Autodesk Inventor part; units mm, degrees
ref_plane "YZ Plane" through (0, 0, 0) normal (1, 0, 0) x (0, 1, 0)
ref_plane "XZ Plane" through (0, 0, 0) normal (0, 1, 0) x (-1, 0, 0)
ref_plane "XY Plane" through (0, 0, 0) normal (0, 0, 1) x (1, 0, 0)
sketch "Skizze10" plane through (0, 0, 0) normal (1, 0, 0) x (0, 1, 0)
  arc A0 (0, -9.6) -> (0, 9.6) centre (0, 0) ccw
  line L0 (0, 0) -> (0, -24.5)
  line L1 (0, 0) -> (0, 24.5)
  line L2 (0, 15.79) -> (24.9524, 15.79) construction
  line L3 (-4.9905, 0) -> (29.9429, 0)
  line L4 (0, -19.91) -> (23.7326, -19.91) construction
  line L5 (0, 24.5) -> (9.5, 24.5)
  line L6 (9.5, 24.5) -> (9.5, 10.2835)
  arc A1 (9.5, -10.2835) -> (9.5, 10.2835) centre (0, 0) ccw
  line L7 (9.5, -10.2835) -> (9.5, -24.5)
  line L8 (0, -24.5) -> (9.5, -24.5)
  point P0 (0, 9.6)
  point P1 (9.5, -19.91)
  point P2 (9.5, 15.79)
  dimension "d79" = 9.6
  dimension "d80" = 24.5
  dimension "d81" = 24.5
  dimension "d82" = 15.79
  dimension "d83" = 19.91
  dimension "d84" = 9.5
  dimension "d85" = 14
extrude "Extrusion9" add sketch "Skizze10" along normal mid plane 8.5 contours A0 L3 A1 L7 L8 L0 | A0 L1 L5 L6 A1 L3
sketch "Skizze11" plane through (0, 0, 0) normal (0, 1, 0) x (-1, 0, 0)
  circle A0 centre (0, -19.91) radius 1.7
  circle A1 centre (0, 15.79) radius 1.7
  line L0 (-4.25, -24.5) -> (-4.25, -10.2835)
  line L1 (0, -32.898) -> (0, 25.888)
  point P0 (0, 0)
  dimension "d88" = 15.79
  dimension "d89" = 19.91
  dimension "d90" = 3.4
  dimension "d91" = 3.4
extrude "Extrusion10" cut sketch "Skizze11" along normal through all
sketch "Skizze12" plane through (0, 0, 0) normal (0, 1, 0) x (-1, 0, 0)
  line L0 (4.25, 9.6) -> (4.25, 24.5)
  line L1 (4.25, 23) -> (-1.05, 23)
  line L2 (-1.05, 23) -> (-1.05, 18.6)
  line L3 (-1.05, 18.6) -> (4.25, 18.6)
  line L4 (4.25, 18.6) -> (4.25, 23)
  line L5 (5.31, 0) -> (-2.11, 0)
  point P0 (0, 0)
  point P1 (4.25, 18.6)
  dimension "d94" = 4.4
  dimension "d95" = 5.3
  dimension "d96" = 18.6
extrude "Extrusion11" cut sketch "Skizze12" along normal blind 3.35
properties part number "Lagerhalter1"
For this review, take the finished solid that the model builds, in its own axes (mm). A direction names the side the tool comes from. Round coordinates to 2 decimals unless told otherwise and drop trailing zeros. Write each loop counter-clockwise with the first axis right and the second up, starting at its lowest first coordinate (ties: lowest second). Pieces come first, ordered by that corner, then holes. Notation, with made-up numbers: M 55,71 L 73,71 A28 ccw 73,89 Z; hole C 54,55.25 d5. An arc over 180 degrees is marked long. Write item = value, one per line. Start each with the question number.
(1) For faces 1 (the face through (-2, 2, 18.6)), 2 (the face through (-4.25, 10, 0)), 3 (the face through (-1, 9.5, 17.5)), 4 (the face through (0, 9.5, -17)), list the 3-axis set-ups (+Z, -Z, +X, -X, +Y, -Y) from which the entire face can be reached by the end or side of a thin tool; tool diameter is ignored.
(2) The part is to be moulded in two halves that separate along X. For faces 5 (the face through (0.2, 4.7, 14.1)), 6 (the face through (-2, 2, 23)), 7 (the face through (4.25, 10, 0)), say which applies: +X half, -X half, draft (parallel to the pull), parting line (faces both ways), or undercut.
(3) For line 1 along X through (y, z) = (3.5, -19.91); line 2 along Z through (x, y) = (0, 3.25); line 3 along Y through (x, z) = (-1.75, -21), list the stretches that pass through material, from the lowest coordinate up.
(4) We need section C-C (z = -19.91). Give the boundary of the cut face in (x, y).
(5) We need section A-A (y = 6.75). Give the boundary of the cut face in (x, z), then the cut area to 3 significant figures.
(6) We need section B-B (x = 0). Give the boundary of the cut face in (y, z), then the cut area to 3 significant figures.
(7) We need section D-D (x = 2.25). Give the boundary of the cut face in (y, z).
(8) Clearance check with flat-ended pins moving along their axes: pin 1 Ø3.5 at (y, z) = (1, 20) entering from -X; pin 2 Ø1.5 at (x, z) = (-1.5, 0.5) entering from -Y; pin 3 Ø2.5 at (x, z) = (2, 18.5) entering from +Y. State where each tip first meets the part, or that it passes through.
Results found:
q1.face_1 = -X, -Y
q1.face_2 = +Z, -Z, -X, +Y, -Y
q1.face_3 = +Z, +X, -X, +Y
q1.face_4 = -Z, +X, -X, +Y
q2.face_5 = undercut
q2.face_6 = draft
q2.face_7 = +X half
q3.line_1 = -4.25 to -1.7, 1.7 to 4.25
q3.line_2 = -24.5 to -21.61, -18.21 to -9.03, 9.03 to 14.09, 17.49 to 18.6, 23 to 24.5
q3.line_3 = 0 to 9.5
q4.outline = M -4.25,0 L -1.7,0 L -1.7,9.5 L -4.25,9.5 Z; M 1.7,0 L 4.25,0 L 4.25,9.5 L 1.7,9.5 Z
q5.outline = M -4.25,-24.5 L 4.25,-24.5 L 4.25,-6.83 L -4.25,-6.83 Z; M -4.25,6.83 L 4.25,6.83 L 4.25,24.5 L -4.25,24.5 Z; hole C 0,-19.91 d3.4; hole C 0,15.79 d3.4
q5.area = 282 mm²
q6.outline = M 0,-24.5 L 9.5,-24.5 L 9.5,-21.61 L 0,-21.61 Z; M 0,-18.21 L 9.5,-18.21 L 9.5,-10.28 A14 ccw 9.5,10.28 L 9.5,14.09 L 0,14.09 L 0,9.6 A9.6 cw 0,-9.6 Z; M 0,17.49 L 9.5,17.49 L 9.5,24.5 L 0,24.5 L 0,23 L 3.35,23 L 3.35,18.6 L 0,18.6 Z
q6.area = 305 mm²
q7.outline = M 0,-24.5 L 9.5,-24.5 L 9.5,-10.28 A14 ccw 9.5,10.28 L 9.5,24.5 L 0,24.5 L 0,9.6 A9.6 cw 0,-9.6 Z
q8.pin_1 = -4.25
q8.pin_2 = 9.52
q8.pin_3 = 9.5
